CAD build for the part. Positions are in the model's coordinates, mm. Round coordinates to 2 decimals unless told otherwise and drop trailing zeros. Loops run counter-clockwise (first coordinate to the right, second up) from the corner with the lowest first, then second, coordinate; pieces in that order, holes last. Notation, with made-up numbers: (86, -38.75) - (96, -38.75) arc R24 ccw to (96, -0.75) - close; hole circle Ø2 at (-8, 41.5). An arc over 180 degrees is marked (long way). Use one line per item in the form item = value.
from build123d import *

# Parameters (mm, degrees)
SKETCH_1_R      = 2
EXTRUDE_1_DEPTH = 1


with BuildPart() as part:
    # Эскиз1 → Бобышка-Вытянуть1 (new body)
    with BuildSketch(Plane.XY):
        with BuildLine():
            Line((5, 0), (20, 0))
            ThreePointArc((20, 0), (23.535533906, -1.464466094), (25, -5))
            ThreePointArc((25, -5), (23.535533906, -8.535533906), (20, -10))
            Line((20, -10), (5, -10))
            ThreePointArc((5, -10), (1.464466094, -8.535533906), (0, -5))
            ThreePointArc((0, -5), (1.464466094, -1.464466094), (5, 0))
        make_face()
        with Locations((5, -5)):
            Circle(SKETCH_1_R, mode=Mode.SUBTRACT)
        with Locations((20, -5)):
            Circle(SKETCH_1_R, mode=Mode.SUBTRACT)
    extrude(amount=EXTRUDE_1_DEPTH)


solid = part.part
1) Slice it at B-B (y = -3.25). Write the cut outline in (x, z).
Report:
outline = (0.32, 0) - (4.03, 0) - (4.03, 1) - (0.32, 1) - close; (5.97, 0) - (19.03, 0) - (19.03, 1) - (5.97, 1) - close; (20.97, 0) - (24.68, 0) - (24.68, 1) - (20.97, 1) - close
2) Slice it at C-C (x = 6). Write the cut outline in (y, z), plus the area to 3 significant figures.
Report:
outline = (-10, 0) - (-6.73, 0) - (-6.73, 1) - (-10, 1) - close; (-3.27, 0) - (0, 0) - (0, 1) - (-3.27, 1) - close
area = 6.54 mm^2
3) Slice it at D-D (x = 21.25). Write the cut outline in (y, z), plus the area to 3 significant figures.
Report:
outline = (-9.84, 0) - (-6.56, 0) - (-6.56, 1) - (-9.84, 1) - close; (-3.44, 0) - (-0.16, 0) - (-0.16, 1) - (-3.44, 1) - close
area = 6.56 mm^2
4) Slice it at A-A (z = 0.5). Write the cut outline in (x, y), plus the area to 3 significant figures.
Report:
outline = (5, -10) - (20, -10) arc R5 ccw to (20, 0) - (5, 0) arc R5 ccw to start; hole circle Ø4 at (5, -5); hole circle Ø4 at (20, -5)
area = 203 mm^2
5) Two-plate mould, pull along X, no slides. Class faces 1 (the cylindrical face through (18.4, -6.2, 0.5)), 2 (the cylindrical face through (3.4, -6.2, 0.5)), 3 (the flat face through (12.6, -10, 0.5)): +X half, -X half, draft (parallel to the pull), parting line (faces both ways), or undercut.
Report:
face_1 = undercut
face_2 = undercut
face_3 = draft
6) Drill centre lines: probe 1 along Y at (x, z) = (20, 0.3); probe 2 along Y at (x, z) = (6.25, 0.35); probe 3 along X at (y, z) = (-3.5, 0.1). Where is each one in solid material? Low to high.
Report:
probe_1 = -10 to -7, -3 to 0
probe_2 = -10 to -6.56, -3.44 to 0
probe_3 = 0.23 to 3.68, 6.32 to 18.68, 21.32 to 24.77
